Verification items for the finished model (mm, model axes). A direction names the side the tool comes from. Coordinates: 2 decimals unless noted, no trailing zeros. Order: outer loops, then holes, each group sorted by start corner. A loop starts at its lowest first (then second) coordinate and runs counter-clockwise, first axis right, second up. Notation, with made-up numbers: (-3.5, 63.5) -> (54.5, 63.5) arc R20 cw to (54.5, 76.5) -> close; hole circle Ø2 at (-28.75, 6). An arc over 180 degrees is marked (long way). Write item = value, one per line. Start each with the question number.
1. Go/stop test with flat-tipped pins: P1, Ø5, axis at y = -15, z = 798.5, coming from the +X side; P2, Ø9.5, axis at y = -19.5, z = 813, coming from the -X side; P3, Ø6, axis at x = 467.5, y = -20, coming from the +Z side. Record where each tip stops, or that it passes through.
2. Set-up check for faces 4 (the flat face through (544, -22, 816)), 5 (the flat face through (291, -22, 778)), 6 (the flat face through (574, -22, 800)), 7 (the flat face through (77.825, -21.874, 800.308)): record each of +Z, -Z, +X, -X, +Y, -Y from which the full face is reachable in a straight line by a thin tool's end or side.
3. Thickness scan on line 1 along Z through (x, y) = (579, -22); line 2 along X through (y, z) = (-13.25, 800); line 3 along Z through (x, y) = (481, -15). Record the ranges inside material, lowest first. Write a range as from..to.
4. Release check for a two-part mould opening along Y. For faces 1 (the flat face through (282, 0, 800)), 2 (the flat face through (31, -13, 800)), 3 (the cylindrical face through (-22, -8, 800)) record: +Y half, -Y half, draft (parallel to the pull), parting line (faces both ways), or undercut.
5. Cross-section at A-A on x = 363.5. Record the cut outline in (y, z), plus the area to 3 significant figures.
from build123d import *

# Parameters (mm, degrees)
F1_DEPTH  = 44
F4_DEPTH  = 18
F5_R      = 4
F6_DEPTH  = 44.001
F7_DEPTH  = 20
F8_R      = 10
F9_DEPTH  = 20
F10_R     = 3
F11_W     = 345
F11_H     = 12
F12_DEPTH = 12


with BuildPart() as f1:
    # F0 (on Front) → F1 (new body)
    with BuildSketch(Plane.XZ):
        with BuildLine():
            Line((594, 822), (0, 822))
            ThreePointArc((0, 822), (-22, 800), (0, 778))
            Line((0, 778), (594, 778))
            Line((594, 778), (594, 822))
        make_face()
    extrude(amount=F1_DEPTH)

    # F3 (on offset) → F4 (cut)
    with BuildSketch(Plane(origin=(0, -13, 0), x_dir=(-1, 0, 0), z_dir=(0, 1, 0))):
        Polygon((-81.7583871512, 778), (22, 778), (22, 822), (-74, 822), align=None)
    extrude(amount=-F4_DEPTH, mode=Mode.SUBTRACT)

    # F5 (on face) → F6 (cut, through all)
    with BuildSketch(Plane(origin=(0, 0, 0), x_dir=(-1, 0, 0), z_dir=(0, 1, 0))):
        with Locations((0, 800)):
            Circle(F5_R)
    extrude(amount=-F6_DEPTH, mode=Mode.SUBTRACT)

    # F5 (on face) → F7 (cut)
    with BuildSketch(Plane(origin=(0, 0, 0), x_dir=(-1, 0, 0), z_dir=(0, 1, 0))):
        with Locations((-218, 800)):
            Circle(F5_R)
        with Locations((-244, 800)):
            Circle(F5_R)
        with Locations((-481, 800)):
            Circle(F5_R)
    extrude(amount=-F7_DEPTH, mode=Mode.SUBTRACT)

    # F8 (on face) → F9 (cut)
    with BuildSketch(Plane.YZ.offset(594)):
        with Locations((-22, 800)):
            Circle(F8_R)
    extrude(amount=-F9_DEPTH, mode=Mode.SUBTRACT)

    # F10
    f10_edges = [f1.edges().sort_by_distance(p)[0] for p in [
        (297, -44, 822),
        (297, 0, 822),
        (594, 0, 800),
        (594, -22, 822),
        (594, -44, 800),
        (594, -22, 778),
    ]]
    fillet(f10_edges, radius=F10_R)

    # F11 (on face) → F12 (cut)
    with BuildSketch(Plane.XY.offset(822)):
        with Locations((371.5, -22)):
            Rectangle(F11_W, F11_H)
    extrude(amount=-F12_DEPTH, mode=Mode.SUBTRACT)


solid = f1.part
Worked out:
q1.P1 = 574
q1.P2 = 74.75
q1.P3 = 810
q2.face_4 = +Z
q2.face_5 = -Z, +X, -X, +Y, -Y
q2.face_6 = +X
q2.face_7 = -Z, -X
q3.line_1 = 778..790, 810..822
q3.line_2 = 77.88..214, 222..240, 248..477, 485..574
q3.line_3 = 778..796, 804..822
q4.face_1 = +Y half
q4.face_2 = undercut
q4.face_3 = draft
q5.outline = (-44, 781) arc R3 ccw to (-41, 778) -> (-3, 778) arc R3 ccw to (0, 781) -> (0, 819) arc R3 ccw to (-3, 822) -> (-16, 822) -> (-16, 810) -> (-28, 810) -> (-28, 822) -> (-41, 822) arc R3 ccw to (-44, 819) -> close
q5.area = 1,780 mm²
